from build123d import *

# Parameters (mm, degrees)
SKETCH_1_R          = 21.25
SKETCH_1_R_2        = 9.25
SKETCH_1_R_3        = 2.5
EXTRUDE_1_DEPTH     = 15
CUT_EXTRUDE_START   = -15
CUT_EXTRUDE_1_DEPTH = 15
SKETCH_3_R          = 1.75
CUT_EXTRUDE_2_DEPTH = 47.280726062
CHAMFER_1_SIZE      = 1
CHAMFER_2_SIZE      = 1
SKETCH_4_R          = 3.5
CUT_EXTRUDE_3_DEPTH = 5


# Read off the part's stored shape, not the designer's step: ｶｯﾄ - 押し出し1
with BuildPart() as part:
    # ｽｹｯﾁ1 → ﾎﾞｽ - 押し出し1 (new body)
    with BuildSketch(Plane.XY):
        Circle(SKETCH_1_R)
        Circle(SKETCH_1_R_2, mode=Mode.SUBTRACT)
        with Locations((15.75, 0)):
            Circle(SKETCH_1_R_3, mode=Mode.SUBTRACT)
        with Locations((13.63990011, -7.875)):
            Circle(SKETCH_1_R_3, mode=Mode.SUBTRACT)
        with Locations((7.875, -13.63990011)):
            Circle(SKETCH_1_R_3, mode=Mode.SUBTRACT)
        with Locations(Location((7.875, 13.63990011, 0), (0, 0, 180))):
            Circle(SKETCH_1_R_3, mode=Mode.SUBTRACT)
        with Locations(Location((13.63990011, 7.875, 0), (0, 0, 180))):
            Circle(SKETCH_1_R_3, mode=Mode.SUBTRACT)
        with Locations(Location((-7.875, -13.63990011, 0), (0, 0, 180))):
            Circle(SKETCH_1_R_3, mode=Mode.SUBTRACT)
        with Locations(Location((-13.63990011, -7.875, 0), (0, 0, 180))):
            Circle(SKETCH_1_R_3, mode=Mode.SUBTRACT)
        with Locations(Location((-15.75, 0, 0), (0, 0, 180))):
            Circle(SKETCH_1_R_3, mode=Mode.SUBTRACT)
        with Locations((-13.63990011, 7.875)):
            Circle(SKETCH_1_R_3, mode=Mode.SUBTRACT)
        with Locations((-7.875, 13.63990011)):
            Circle(SKETCH_1_R_3, mode=Mode.SUBTRACT)
    extrude(amount=EXTRUDE_1_DEPTH)

    # ｶｯﾄ - 押し出し1 outline → ｶｯﾄ - 押し出し1 (cut)
    with BuildSketch(Plane.XY.offset(15).offset(CUT_EXTRUDE_START)):
        with BuildLine():
            Line((-9.231832093, 19.13990011), (9.231832093, 19.13990011))
            ThreePointArc((9.231832093, 19.13990011), (0, 21.25), (-9.231832093, 19.13990011))
        make_face()
        with BuildLine():
            Line((9.231832093, -19.13990011), (-9.231832093, -19.13990011))
            ThreePointArc((-9.231832093, -19.13990011), (0, -21.25), (9.231832093, -19.13990011))
        make_face()
    extrude(amount=CUT_EXTRUDE_1_DEPTH, mode=Mode.SUBTRACT)

    # ｽｹｯﾁ3 → ｶｯﾄ - 押し出し2 (cut, through all)
    with BuildSketch(Plane(origin=(0, 19.13990011, 0), x_dir=(1, 0, 0), z_dir=(0, 1, 0))):
        with Locations(Location((0, -7.5, 0), (0, 0, 270))):
            Circle(SKETCH_3_R)
    extrude(amount=-CUT_EXTRUDE_2_DEPTH, mode=Mode.SUBTRACT)

    # 面取り1
    chamfer_1_edges = [part.edges().sort_by_distance(p)[0] for p in [
        (10.375, 13.63990011, 0),
        (10.375, 13.63990011, 15),
        (11.13990011, -7.875, 0),
        (11.13990011, -7.875, 15),
        (5.375, -13.63990011, 0),
        (5.375, -13.63990011, 15),
        (16.13990011, 7.875, 0),
        (16.13990011, 7.875, 15),
        (-5.375, -13.63990011, 0),
        (-5.375, -13.63990011, 15),
        (-11.13990011, -7.875, 0),
        (-11.13990011, -7.875, 15),
        (-13.25, 0, 0),
        (-13.25, 0, 15),
        (-16.13990011, 7.875, 0),
        (-16.13990011, 7.875, 15),
        (-10.375, 13.63990011, 0),
        (-10.375, 13.63990011, 15),
        (13.25, 0, 0),
        (13.25, 0, 15),
    ]]
    chamfer(chamfer_1_edges, length=CHAMFER_1_SIZE)

    # 面取り2
    chamfer_2_edges = [part.edges().sort_by_distance(p)[0] for p in [
        (-21.25, 0, 15),
        (21.25, 0, 15),
        (-21.25, 0, 0),
        (21.25, 0, 0),
        (0, 19.13990011, 0),
        (0, -19.13990011, 0),
        (0, -19.13990011, 15),
        (0, 19.13990011, 15),
    ]]
    chamfer(chamfer_2_edges, length=CHAMFER_2_SIZE)

    # ｽｹｯﾁ4 → ｶｯﾄ - 押し出し3 (cut)
    with BuildSketch(Plane(origin=(0, 19.13990011, 0), x_dir=(1, 0, 0), z_dir=(0, 1, 0))):
        with Locations(Location((0, -7.5, 0), (0, 0, 270))):
            Circle(SKETCH_4_R)
    extrude(amount=-CUT_EXTRUDE_3_DEPTH, mode=Mode.SUBTRACT)


solid = part.part
Verification items for the finished model (mm, model axes). Coordinates: 2 decimals unless noted, no trailing zeros. Order: outer loops, then holes, each group sorted by start corner. A loop starts at its lowest first (then second) coordinate and runs counter-clockwise, first axis right, second up. Notation, with made-up numbers: (-22, 81) -> (-3, 81) arc R11 cw to (-3, 85) -> close; hole circle Ø5 at (84.25, 26). An arc over 180 degrees is marked (long way). Use CSV: the item, a comma, the result in double quotes. Start each with the question number.
Q1. Depth check by flat-ended pin: P1, Ø1, axis at x = 14.5, z = 10.5, coming from the -Y side; P2, Ø6, axis at x = 15.75, y = 0, coming from the +Z side; P3, Ø12, axis at x = 11.5, y = -3, coming from the -Z side; P4, Ø6.5, axis at x = 7.88, y = -13.64, coming from the -Z side (3 decimals). Enter the tip coordinate at first touch or a pass-through.
Q2. Section check B-B, the plane z = 7.5. Give the number of separate pieces and of enclosed holes in the cut face, and give its area (3 significant figures).
Q3. Section check A-A, the plane y = 0. Record the cut outline in (x, z), and give its area (3 significant figures).
Q4. Section check C-C, the plane x = 0. Record the cut outline in (y, z).
Q5. Thickness scan on line 1 along Y through (x, z) = (-0.5, 3); line 2 along Y through (x, z) = (15.75, 6.5); line 3 along X through (y, z) = (7, 7.5). Record the ranges inside material, lowest first.
Q6. Draft check along Y on faces 1 (the flat face through (-0.13, 18.63, 14.51)), 2 (the flat face through (-5, 8, 15)), 3 (the flat face through (0.13, -18.63, 14.51)), 4 (the cylindrical face through (-10.26, -14.39, 7.41)). Enter one of: +Y half, -Y half, draft (parallel to the pull), parting line (faces both ways), or undercut.
Returned:
1,P1,"stops at y = -15.99"
1,P2,"stops at z = 14.5"
1,P3,"stops at z = 0"
1,P4,"stops at z = 0.245"
2,separate pieces,"2"
2,enclosed holes,"10"
2,area,"814 mm^2"
3,outline,"(-21.25, 1) -> (-20.25, 0) -> (-19.25, 0) -> (-18.25, 1) -> (-18.25, 14) -> (-19.25, 15) -> (-20.25, 15) -> (-21.25, 14) -> close; (-13.25, 1) -> (-12.25, 0) -> (-9.25, 0) -> (-9.25, 15) -> (-12.25, 15) -> (-13.25, 14) -> close; (9.25, 0) -> (12.25, 0) -> (13.25, 1) -> (13.25, 14) -> (12.25, 15) -> (9.25, 15) -> close; (18.25, 1) -> (19.25, 0) -> (20.25, 0) -> (21.25, 1) -> (21.25, 14) -> (20.25, 15) -> (19.25, 15) -> (18.25, 14) -> close"
3,area,"204 mm^2"
4,outline,"(-19.14, 1) -> (-18.14, 0) -> (-9.25, 0) -> (-9.25, 5.75) -> (-19.14, 5.75) -> close; (-19.14, 9.25) -> (-9.25, 9.25) -> (-9.25, 15) -> (-18.14, 15) -> (-19.14, 14) -> close; (9.25, 0) -> (18.14, 0) -> (19.14, 1) -> (19.14, 4) -> (14.14, 4) -> (14.14, 5.75) -> (9.25, 5.75) -> close; (9.25, 9.25) -> (14.14, 9.25) -> (14.14, 11) -> (19.14, 11) -> (19.14, 14) -> (18.14, 15) -> (9.25, 15) -> close"
5,line 1,"y = -19.14 to -9.24, 9.24 to 19.14"
5,line 2,"y = -14.27 to -9.22, -6.53 to -2.5, 2.5 to 6.53, 9.22 to 14.27"
5,line 3,"x = -20.06 to -15.98, -11.3 to -6.05, 6.05 to 11.3, 15.98 to 20.06"
6,face 1,"+Y half"
6,face 2,"draft"
6,face 3,"-Y half"
6,face 4,"undercut"
